```python
from build123d import *

# Parameters (mm, degrees)
SKETCH_1_W          = 140
SKETCH_1_H          = 80
SKETCH_1_R          = 1.6
EXTRUDE_1_DEPTH     = 3
SKETCH_2_R          = 1.6
CUT_EXTRUDE_1_DEPTH = 10
SKETCH_3_W          = 55
SKETCH_3_H          = 30
CUT_EXTRUDE_2_DEPTH = 10
FILLET_1_R          = 5
FILLET_2_R          = 10
SKETCH_4_R          = 1.6
CUT_EXTRUDE_3_DEPTH = 10
SKETCH_6_W          = 20
SKETCH_6_H          = 25
EXTRUDE_2_DEPTH     = 3
SKETCH_7_R          = 1.6
CUT_EXTRUDE_5_DEPTH = 4
FILLET_3_R          = 5


with BuildPart() as part:
    # 草图1 → 凸台-拉伸1 (new body)
    with BuildSketch(Plane.XY):
        Rectangle(SKETCH_1_W, SKETCH_1_H)
        with Locations((19.25, 33.341978046)):
            Circle(SKETCH_1_R, mode=Mode.SUBTRACT)
        with Locations((38.5, 0)):
            Circle(SKETCH_1_R, mode=Mode.SUBTRACT)
        with Locations((19.25, -33.341978046)):
            Circle(SKETCH_1_R, mode=Mode.SUBTRACT)
        with Locations((-19.25, -33.341978046)):
            Circle(SKETCH_1_R, mode=Mode.SUBTRACT)
        with Locations((-38.5, 0)):
            Circle(SKETCH_1_R, mode=Mode.SUBTRACT)
        with Locations((-19.25, 33.341978046)):
            Circle(SKETCH_1_R, mode=Mode.SUBTRACT)
    extrude(amount=EXTRUDE_1_DEPTH)

    # 草图2 → 切除-拉伸1 (cut)
    with BuildSketch(Plane.XY.offset(3)):
        with Locations((0, 25)):
            Circle(SKETCH_2_R)
        with Locations((-60, 25)):
            Circle(SKETCH_2_R)
        with Locations((60, 25)):
            Circle(SKETCH_2_R)
        with Locations((60, -25)):
            Circle(SKETCH_2_R)
        with Locations((-60, -25)):
            Circle(SKETCH_2_R)
        with Locations((0, -25)):
            Circle(SKETCH_2_R)
    extrude(amount=-CUT_EXTRUDE_1_DEPTH, mode=Mode.SUBTRACT)

    # 草图3 → 切除-拉伸2 (cut)
    with BuildSketch(Plane.XY.offset(3)):
        Rectangle(SKETCH_3_W, SKETCH_3_H)
    extrude(amount=-CUT_EXTRUDE_2_DEPTH, mode=Mode.SUBTRACT)

    # 圆角1
    fillet_1_edges = [part.edges().sort_by_distance(p)[0] for p in [
        (27.5, 15, 1.5),
        (27.5, -15, 1.5),
        (-27.5, -15, 1.5),
        (-27.5, 15, 1.5),
    ]]
    fillet(fillet_1_edges, radius=FILLET_1_R)

    # 圆角2
    fillet_2_edges = [part.edges().sort_by_distance(p)[0] for p in [
        (70, -40, 1.5),
        (-70, -40, 1.5),
        (-70, 40, 1.5),
        (70, 40, 1.5),
    ]]
    fillet(fillet_2_edges, radius=FILLET_2_R)

    # 草图4 → 切除-拉伸3 (cut)
    with BuildSketch(Plane.XY.offset(3)):
        with Locations((-50, 25)):
            Circle(SKETCH_4_R)
        with Locations((-50, -25)):
            Circle(SKETCH_4_R)
        with Locations((50, -25)):
            Circle(SKETCH_4_R)
        with Locations((50, 25)):
            Circle(SKETCH_4_R)
    extrude(amount=-CUT_EXTRUDE_3_DEPTH, mode=Mode.SUBTRACT)

    # 草图6 → 凸台-拉伸2 (add)
    with BuildSketch(Plane.XY.offset(3)):
        with Locations((0, -52.5)):
            Rectangle(SKETCH_6_W, SKETCH_6_H)
    extrude(amount=-EXTRUDE_2_DEPTH)

    # 草图7 → 切除-拉伸5 (cut, through all)
    with BuildSketch(Plane.XY.offset(3)):
        with Locations((0, -45)):
            Circle(SKETCH_7_R)
        with Locations((0, -55)):
            Circle(SKETCH_7_R)
    extrude(amount=-CUT_EXTRUDE_5_DEPTH, mode=Mode.SUBTRACT)

    # 圆角3
    fillet_3_edges = [part.edges().sort_by_distance(p)[0] for p in [
        (-10, -40, 1.5),
        (10, -40, 1.5),
        (10, -65, 1.5),
        (-10, -65, 1.5),
    ]]
    fillet(fillet_3_edges, radius=FILLET_3_R)


solid = part.part
```
Part model, mm, in its own coordinate system. A direction names the side the tool comes from. Coordinates: 2 decimals unless noted, no trailing zeros. Order: outer loops, then holes, each group sorted by start corner. A loop starts at its lowest first (then second) coordinate and runs counter-clockwise, first axis right, second up. Notation, with made-up numbers: (-26, -22) - (17, -22) arc R23 ccw to (17, 14) - close; hole circle Ø6 at (83.25, 16.5). An arc over 180 degrees is marked (long way). Return JSON: item names as keys, results as strings. Group by question number.
Item 1: Which spindle directions (+Z, -Z, +X, -X, +Y, -Y) get a long thin tool onto all of the face, cutting with end or side? Do faces 4 (the face through (-12, -41, 1)), 5 (the face through (37, -40, 1)), 6 (the face through (27.5, 0, 2)). Say none if no direction does.
Item 2: Pin check, flat tips, straight feed: pin 1 (1.9 mm diameter, centred on x = 0, y = -25, fed in from +Z); pin 2 (0.9 mm diameter, centred on x = -37.5, z = 2, fed in from -Y); pin 3 (1.5 mm diameter, centred on y = -52.5, z = 2, fed in from +X); pin 4 (0.9 mm diameter, centred on y = -50.5, z = 2, fed in from -X). Stop position of each tip, or through.
Item 3: Cut at C-C (x = 0). List the corners of the cut face in (y, z).
Item 4: Pull direction Y, two halves, no side cores. Call faces 1 (the face through (-10, -53, 2)), 2 (the face through (26, -13.57, 1.48)), 3 (the face through (8, -64, 1)): pulls with the +Y half, pulls with the -Y half, needs draft (parallel to the pull), parting line crosses it, or undercut.
Item 5: Drill centre lines: probe 1 along Y at (x, z) = (-19.25, 1.5); probe 2 along Y at (x, z) = (0, 1.2); probe 3 along Y at (x, z) = (17.5, 0.9). Where is each one in solid material? Low to high. Write a range as from..to.
Item 6: Cut at B-B (x = 19.25). List the corners of the cut face in (y, z), plus the area to 3 significant figures.
Item 7: Cut at A-A (y = -55). List the corners of the cut face in (x, z), plus the area to 3 significant figures.
Item 8: Cut at D-D (y = 25). List the corners of the cut face in (x, z), plus the area to 3 significant figures.
Check values:
{
 "1": {"face 4": "+Z, -Z, -X, -Y", "face 5": "+Z, -Z, +X, -Y", "face 6": "+Z, -Z"},
 "2": {"pin 1": "passes through", "pin 2": "stops at y = -40", "pin 3": "stops at x = 10", "pin 4": "stops at x = -10"},
 "3": {"outline": "(-65, 0) - (-56.6, 0) - (-56.6, 3) - (-65, 3) - close; (-53.4, 0) - (-46.6, 0) - (-46.6, 3) - (-53.4, 3) - close; (-43.4, 0) - (-26.6, 0) - (-26.6, 3) - (-43.4, 3) - close; (-23.4, 0) - (-15, 0) - (-15, 3) - (-23.4, 3) - close; (15, 0) - (23.4, 0) - (23.4, 3) - (15, 3) - close; (26.6, 0) - (40, 0) - (40, 3) - (26.6, 3) - close"},
 "4": {"face 1": "needs draft", "face 2": "undercut", "face 3": "pulls with the -Y half"},
 "5": {"probe 1": "y = -40..-34.94, -31.74..-15, 15..31.74, 34.94..40", "probe 2": "y = -65..-56.6, -53.4..-46.6, -43.4..-26.6, -23.4..-15, 15..23.4, 26.6..40", "probe 3": "y = -40..-15, 15..40"},
 "6": {"outline": "(-40, 0) - (-34.94, 0) - (-34.94, 3) - (-40, 3) - close; (-31.74, 0) - (-15, 0) - (-15, 3) - (-31.74, 3) - close; (15, 0) - (31.74, 0) - (31.74, 3) - (15, 3) - close; (34.94, 0) - (40, 0) - (40, 3) - (34.94, 3) - close", "area": "131 mm2"},
 "7": {"outline": "(-10, 0) - (-1.6, 0) - (-1.6, 3) - (-10, 3) - close; (1.6, 0) - (10, 0) - (10, 3) - (1.6, 3) - close", "area": "50.4 mm2"},
 "8": {"outline": "(-70, 0) - (-61.6, 0) - (-61.6, 3) - (-70, 3) - close; (-58.4, 0) - (-51.6, 0) - (-51.6, 3) - (-58.4, 3) - close; (-48.4, 0) - (-1.6, 0) - (-1.6, 3) - (-48.4, 3) - close; (1.6, 0) - (48.4, 0) - (48.4, 3) - (1.6, 3) - close; (51.6, 0) - (58.4, 0) - (58.4, 3) - (51.6, 3) - close; (61.6, 0) - (70, 0) - (70, 3) - (61.6, 3) - close", "area": "372 mm2"}
}
